Here's how the part is built. I have some questions about the finished solid (model axes, mm). Face numbers are marked on the shaded views. A direction names the side the tool comes from. Coordinates: 2 decimals unless noted, no trailing zeros. Order: outer loops, then holes, each group sorted by start corner. A loop starts at its lowest first (then second) coordinate and runs counter-clockwise, first axis right, second up. Notation, with made-up numbers: (42, -5) - (57, -5) arc R14 cw to (57, 22) - close; hole circle Ø1 at (-35.75, 9). An arc over 180 degrees is marked (long way). Answer in a Markdown table with one row per item. Add a question column.
Item 1: I want a section at B-B (x = -166.5). Please give me the cut outline in (y, z).
Item 2: I want a section at D-D (z = -34.5). Please give me the cut outline in (x, y), plus the area to 3 significant figures.
Item 3: Thinking about a two-plate mould opening in Z: for the marked faces 1, 2 and 3, which applies, +Z half, -Z half, draft (parallel to the pull), parting line (faces both ways), or undercut?
Item 4: I want a section at C-C (y = -67.1). Please give me the cut outline in (x, z).
Item 5: On a 3-axis mill with a long thin cutter (end or side, diameter ignored), from which of +Z, -Z, +X, -X, +Y, -Y can I reach the whole of each face in a straight line? I mean the marked faces 4, 5, 6 and 7. Say none if no direction works.
Item 6: If I drill on line 1 along Y through (x, z) = (-161, -35); line 2 along X through (y, z) = (-67.1, -35.5); line 3 along Y through (x, z) = (-165, -33.25), over which ranges is the centre line in solid material (lowest first)? Write a range as from..to.
Item 7: Will these pins go through, and if not, where does the flat tip stop? pin 1 Ø0.7 at (y, z) = (-67.5, -41) entering from +X; pin 2 Ø1.1 at (x, y) = (-161, -67) entering from -Z; pin 3 Ø1.6 at (x, z) = (-158.5, -38.5) entering from -Y; pin 4 Ø6 at (x, z) = (-163.5, -32.5) entering from -Y.
Item 8: I want a section at A-A (z = -39.75). Please give me the cut outline in (x, y), plus the area to 3 significant figures.
```python
from build123d import *

# Parameters (mm, degrees)
BOSS_EXTRUDE1_DEPTH = 1.5
BOSS_EXTRUDE2_DEPTH = 10.18
SKETCH2_W           = 2.5
SKETCH2_H           = 0.9
SKETCH2_W_2         = 0.1
BOSS_EXTRUDE3_DEPTH = 1


with BuildPart() as part:
    # Sketch1 → Boss-Extrude1 (new body)
    with BuildSketch(Plane(origin=(-157.854562907, 0, 0), x_dir=(0, 0, -1), z_dir=(1, 0, 0))):
        with BuildLine():
            Line((30.880645232, -65.123367101), (30.880645232, -66.623367101))
            Line((30.880645232, -66.623367101), (33.480645232, -66.623367101))
            Line((33.480645232, -66.623367101), (33.480645232, -70.636755446))
            ThreePointArc((33.480645232, -70.636755446), (33.551588291, -70.599584622), (33.630645232, -70.586755446))
            Line((33.630645232, -70.586755446), (40.030645232, -70.586755446))
            ThreePointArc((40.030645232, -70.586755446), (40.109702174, -70.599584622), (40.180645232, -70.636755446))
            Line((40.180645232, -70.636755446), (40.180645232, -70.412491378))
            ThreePointArc((40.180645232, -70.412491378), (40.106741123, -70.393236094), (40.030645232, -70.386755446))
            Line((40.030645232, -70.386755446), (36.830645232, -70.386755446))
            Line((36.830645232, -70.386755446), (36.830645232, -66.623367101))
            Line((36.830645232, -66.623367101), (38.630645232, -66.623367101))
            ThreePointArc((38.630645232, -66.623367101), (39.576456801, -66.921353611), (40.180645232, -67.707681676))
            Line((40.180645232, -67.707681676), (40.180645232, -66.623367101))
            Line((40.180645232, -66.623367101), (42.780645232, -66.623367101))
            Line((42.780645232, -66.623367101), (42.780645232, -65.123367101))
            Line((42.780645232, -65.123367101), (30.880645232, -65.123367101))
        make_face()
    extrude(amount=-BOSS_EXTRUDE1_DEPTH)

    # Sketch1<3> → Boss-Extrude2 (add)
    with BuildSketch(Plane(origin=(-157.854562907, 0, 0), x_dir=(0, 0, -1), z_dir=(1, 0, 0))):
        Polygon((30.880645232, -65.123367101), (30.880645232, -66.623367101), (33.380645232, -66.623367101), (33.480645232, -66.623367101), (38.630645232, -66.623367101), (40.180645232, -66.623367101), (40.280645232, -66.623367101), (42.780645232, -66.623367101), (42.780645232, -65.123367101), align=None)
    extrude(amount=-BOSS_EXTRUDE2_DEPTH)

    # Sketch2 → Boss-Extrude3 (add)
    with BuildSketch(Plane.XZ.offset(66.623367101)):
        Polygon((-167.184562907, -32.480645232), (-167.184562907, -34.980645232), (-166.184562907, -34.980645232), (-166.184562907, -33.480645232), (-164.684562907, -33.480645232), (-164.684562907, -32.480645232), align=None)
        with Locations((-160.704562907, -40.730645232)):
            Rectangle(SKETCH2_W, SKETCH2_H)
        with Locations((-159.404562907, -40.730645232)):
            Rectangle(SKETCH2_W_2, SKETCH2_H)
    extrude(amount=BOSS_EXTRUDE3_DEPTH)


solid = part.part
```
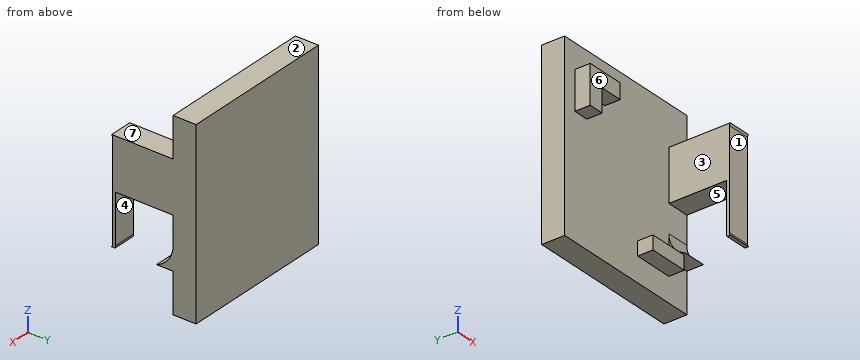
Values follow:
| question | item | result |
|---|---|---|
| 1 | outline | (-67.62, -34.98) - (-66.62, -34.98) - (-66.62, -42.78) - (-65.12, -42.78) - (-65.12, -30.88) - (-66.62, -30.88) - (-66.62, -32.48) - (-67.62, -32.48) - close |
| 2 | outline | (-168.03, -66.62) - (-167.18, -66.62) - (-167.18, -67.62) - (-166.18, -67.62) - (-166.18, -66.62) - (-159.35, -66.62) - (-159.35, -70.59) - (-157.85, -70.59) - (-157.85, -65.12) - (-168.03, -65.12) - close |
| 2 | area | 22.2 mm^2 |
| 3 | face 1 | undercut |
| 3 | face 2 | +Z half |
| 3 | face 3 | draft |
| 4 | outline | (-167.18, -34.98) - (-166.18, -34.98) - (-166.18, -33.48) - (-164.68, -33.48) - (-164.68, -32.48) - (-167.18, -32.48) - close; (-161.95, -41.18) - (-159.35, -41.18) - (-159.35, -40.28) - (-161.95, -40.28) - close; (-159.35, -40.18) - (-157.85, -40.18) - (-157.85, -39.79) - (-159.35, -39.79) - close; (-159.35, -36.83) - (-157.85, -36.83) - (-157.85, -33.48) - (-159.35, -33.48) - close |
| 5 | face 4 | -Z, +X, -X |
| 5 | face 5 | +X, -X |
| 5 | face 6 | +Z, -Z, -X, -Y |
| 5 | face 7 | +Z, +X, -Y |
| 6 | line 1 | y = -66.62..-65.12 |
| 6 | line 2 | x = -159.35..-157.85 |
| 6 | line 3 | y = -67.62..-65.12 |
| 7 | pin 1 | stops at x = -159.35 |
| 7 | pin 2 | stops at z = -42.78 |
| 7 | pin 3 | stops at y = -70.59 |
| 7 | pin 4 | stops at y = -67.62 |
| 8 | outline | (-168.03, -66.62) - (-159.35, -66.62) - (-159.35, -67.06) - (-157.85, -67.06) - (-157.85, -65.12) - (-168.03, -65.12) - close; (-159.35, -70.59) - (-157.85, -70.59) - (-157.85, -70.39) - (-159.35, -70.39) - close |
| 8 | area | 16.2 mm^2 |
